```python
from build123d import *

# Parameters (mm, degrees)
SKETCH1_W            = 80
SKETCH1_H            = 80
BOSS_EXTRUDE1_DEPTH  = 33
SKETCH2_R            = 4
CUT_EXTRUDE1_DEPTH   = 33
LPATTERN1_COUNT      = 8
LPATTERN1_PITCH      = 10
LPATTERN1_COUNT_DIR2 = 7
LPATTERN1_PITCH_DIR2 = 10


with BuildPart() as part:
    # Sketch1 → Boss-Extrude1 (new body)
    with BuildSketch(Plane.XY):
        with Locations((-28.209195922, -3.087248322)):
            Rectangle(SKETCH1_W, SKETCH1_H)
    extrude(amount=BOSS_EXTRUDE1_DEPTH)

    # Sketch2 → Cut-Extrude1 (cut)
    with BuildSketch(Plane.XY.offset(33)):
        with Locations((-61.00943387, 31.665384742)):
            Circle(SKETCH2_R)
    cut_extrude1 = extrude(amount=-CUT_EXTRUDE1_DEPTH, mode=Mode.SUBTRACT)

    # LPattern1: Cut-Extrude1 8 × 7
    with Locations(*[(j * LPATTERN1_PITCH_DIR2, -i * LPATTERN1_PITCH, 0) for i in range(LPATTERN1_COUNT) for j in range(LPATTERN1_COUNT_DIR2) if (i, j) != (0, 0)]):
        add(cut_extrude1, mode=Mode.SUBTRACT)


solid = part.part
```
Geometry check sheet. Reference: the model listing, model coordinates, mm. Round coordinates to 2 decimals unless told otherwise and drop trailing zeros. Return JSON: item names as keys, results as strings. Group by question number.
Q1. Gauge pin test, flat end, axial feed: pin 1 (3 mm diameter, centred on x = -2.5, y = -7.5, fed in from +Z). Record the tip position at first contact, or that the pin passes through.
Q2. Release check for a two-part mould opening along Y. For faces 1 (the cylindrical face through (-1.88, -32.24, 16.73)), 2 (the flat face through (-29, -43.087, 16)) record: released by +Y, released by -Y, zero draft, split by the parting line, or undercut.
Q3. Section check A-A, the plane x = -34. Count the separate pieces of the cut face and the enclosed holes in it, plus the area to 3 significant figures.
Numbers:
{
 "1": {"pin 1": "through"},
 "2": {"face 1": "undercut", "face 2": "released by -Y"},
 "3": {"separate pieces": "9", "enclosed holes": "0", "area": "1,240 mm^2"}
}
